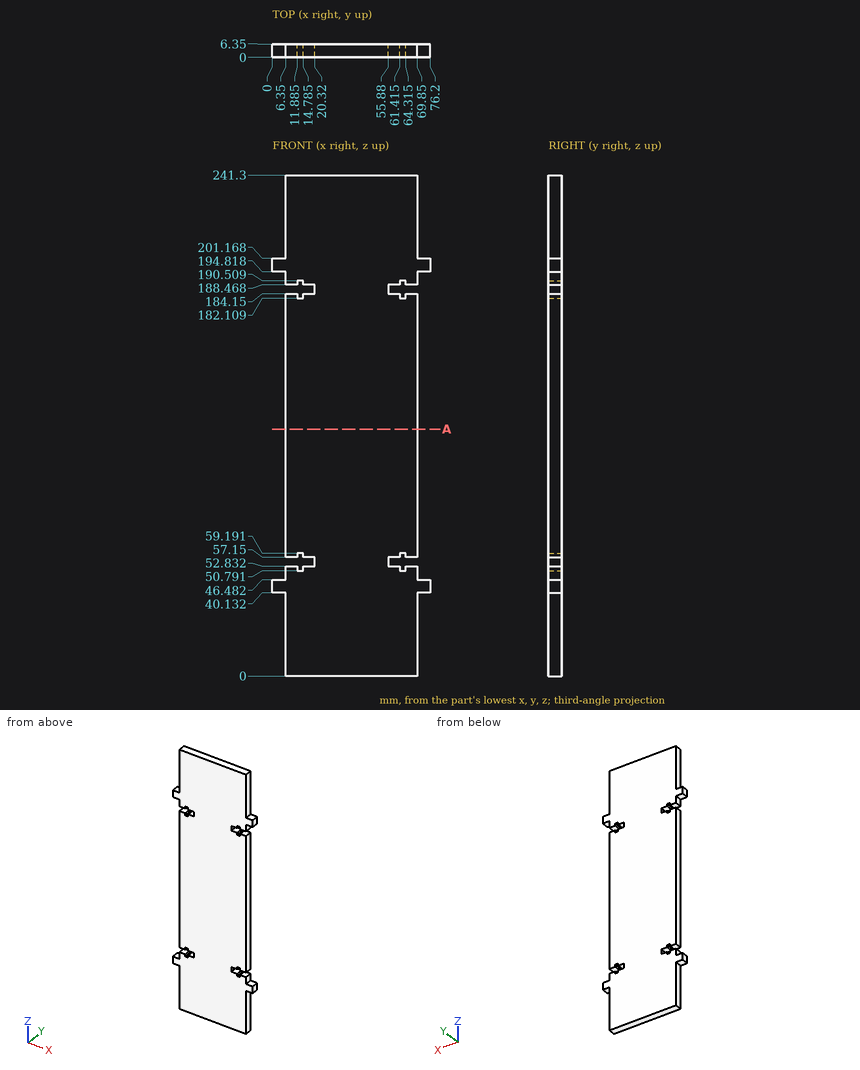
Design review of the part shown in the three views and the two pictorial views. Dimensions are in mm from the part's minimum x, y and z. Give positions to 0.01 mm unless a question says otherwise; leave off trailing zeros. Loops run counter-clockwise (first coordinate to the right, second up) from the corner with the lowest first, then second, coordinate; pieces in that order, holes last. Notation, with made-up numbers: M -15,46 L -3,46 A13 ccw -3,62 Z; hole C -15.5,50 d4. An arc over 180 degrees is marked long. Write item = value, one per line.
Q1. Insertion check: pin 1 (2 mm diameter, centred on y = 3, z = 189, fed in from +X); pin 2 (1.3 mm diameter, centred on y = 4.5, z = 55, fed in from +X); pin 3 (2 mm diameter, centred on y = 1.5, z = 29, fed in from -X). Each pin has a flat end and moves straight along its axis. Give the tip position at first contact, or say it passes through.
Output values:
pin_1 = 69.85
pin_2 = 55.88
pin_3 = 6.35
Q2. To check wall thickness, follow line 1 (Z direction, x = 59.5, y = 5.5); line 2 (X direction, y = 4.5, z = 190) (3 decimals); line 3 (Z direction, x = 14.5, y = 0.5). State the ranges of each line that lie inside material, in increasing order. Write a range as [from, to].
Output values:
line_1 = [0, 52.83], [57.15, 184.15], [188.47, 241.3]
line_2 = [6.35, 11.885], [14.785, 61.415], [64.315, 69.85]
line_3 = [0, 50.79], [59.19, 182.11], [190.51, 241.3]
Q3. We need section A-A (z = 119). Give the boundary of the cut face in (x, y).
Output values:
outline = M 6.35,0 L 69.85,0 L 69.85,6.35 L 6.35,6.35 Z
